Can you work these out from the model? Positions are in its coordinate system, mm. A direction names the side the tool comes from. Round coordinates to 2 decimals unless told otherwise and drop trailing zeros. Loops run counter-clockwise (first coordinate to the right, second up) from the corner with the lowest first, then second, coordinate; pieces in that order, holes last. Notation, with made-up numbers: M -20,-38.75 L 29,-38.75 A10 cw 29,-28.75 Z; hole C 77,27 d3. An arc over 180 degrees is marked long. Return JSON: item names as keys, results as strings.
```python
from build123d import *

# Parameters (mm, degrees)
SKETCH2_R                             = 14
SKETCH2_R_2                           = 11
BOSS_EXTRUDE7_DEPTH                   = 15
SKETCH2_12_R                          = 11
BOSS_EXTRUDE10_DEPTH                  = 3
SKETCH2_9_R                           = 14
SKETCH2_9_R_2                         = 11
BOSS_EXTRUDE8_DEPTH                   = 20
SKETCH2_11_R                          = 11
SKETCH2_11_R_2                        = 8.75
BOSS_EXTRUDE9_DEPTH                   = 12.5
BOSS_EXTRUDE11_REACH                  = 119.015
BOSS_EXTRUDE11_END_RADIUS             = 14
BOSS_EXTRUDE11_DIRECTION_2_REACH      = 119.015
BOSS_EXTRUDE11_DIRECTION_2_END_RADIUS = 14
CUT_EXTRUDE6_DEPTH                    = 1.1
SKETCH13_R                            = 1.15
CUT_EXTRUDE7_DEPTH                    = 3
BOSS_EXTRUDE12_REACH                  = 119.21
SKETCH15_W                            = 3
SKETCH15_H                            = 9.5
FILLET1_R                             = 2


with BuildPart() as part:
    # Sketch2 → Boss-Extrude7 (new body)
    with BuildSketch(Plane(origin=(0, 0, 0), x_dir=(1, 0, 0), z_dir=(0, 1, 0))):
        with Locations(Location((-50, 3.220631283, 0), (0, 0, 270))):
            Circle(SKETCH2_R)
        with Locations(Location((-50, 3.220631283, 0), (0, 0, 270))):
            Circle(SKETCH2_R_2, mode=Mode.SUBTRACT)
    extrude(amount=BOSS_EXTRUDE7_DEPTH)

    # Sketch2<12> → Boss-Extrude10 (add)
    with BuildSketch(Plane(origin=(0, 0, 0), x_dir=(1, 0, 0), z_dir=(0, 1, 0))):
        with Locations(Location((-50, 3.220631283, 0), (0, 0, 270))):
            Circle(SKETCH2_12_R)
    extrude(amount=BOSS_EXTRUDE10_DEPTH)


with BuildPart() as body_2:
    # Sketch2<9> → Boss-Extrude8 (new body)
    with BuildSketch(Plane(origin=(0, 0, 0), x_dir=(1, 0, 0), z_dir=(0, 1, 0))):
        with Locations(Location((100, 3.220631283, 0), (0, 0, 270))):
            Circle(SKETCH2_9_R)
        with Locations(Location((100, 3.220631283, 0), (0, 0, 270))):
            Circle(SKETCH2_9_R_2, mode=Mode.SUBTRACT)
    extrude(amount=BOSS_EXTRUDE8_DEPTH)

    # Sketch2<11> → Boss-Extrude9 (add)
    with BuildSketch(Plane(origin=(0, 0, 0), x_dir=(1, 0, 0), z_dir=(0, 1, 0))):
        with Locations(Location((100, 3.220631283, 0), (0, 0, 270))):
            Circle(SKETCH2_11_R)
        with Locations(Location((100, 3.220631283, 0), (0, 0, 270))):
            Circle(SKETCH2_11_R_2, mode=Mode.SUBTRACT)
    extrude(amount=BOSS_EXTRUDE9_DEPTH)


    add(part.part)  # Boss-Extrude11 merges part
    # Boss-Extrude11: up to this cylinder (the profile starts outside it)
    boss_extrude11_end = Plane(origin=(-50, 0.212132, -3.220631283), z_dir=(0, -1, 0)) * Cylinder(BOSS_EXTRUDE11_END_RADIUS, 267.03, mode=Mode.PRIVATE)
    # Sketch3 → Boss-Extrude11 (add, up to the surface)
    with BuildSketch(Plane(origin=(0, 0, 0), x_dir=(0, 0, -1), z_dir=(1, 0, 0)), mode=Mode.PRIVATE) as boss_extrude11_sk1:
        Polygon((10.720631283, 0), (10.720631283, 15), (-4.279368717, 15), (-4.279368717, 0), (-1.279368717, 0), (-1.279368717, 12), (7.720631283, 12), (7.720631283, 0), align=None)
    boss_extrude11_tool1 = extrude(boss_extrude11_sk1.sketch, amount=-BOSS_EXTRUDE11_REACH, mode=Mode.PRIVATE) - boss_extrude11_end
    add(boss_extrude11_tool1.solids().sort_by_distance((0, 0.212132, -9.220631))[0])

    # Boss-Extrude11 direction 2: up to this cylinder (the profile starts outside it)
    boss_extrude11_direction_2_end = Plane(origin=(100, 0.212132, -3.220631283), z_dir=(0, -1, 0)) * Cylinder(BOSS_EXTRUDE11_DIRECTION_2_END_RADIUS, 267.03, mode=Mode.PRIVATE)
    # Sketch3 → Boss-Extrude11 direction 2 (add, up to the surface)
    with BuildSketch(Plane(origin=(0, 0, 0), x_dir=(0, 0, -1), z_dir=(1, 0, 0)), mode=Mode.PRIVATE) as boss_extrude11_direction_2_sk1:
        Polygon((10.720631283, 0), (10.720631283, 15), (-4.279368717, 15), (-4.279368717, 0), (-1.279368717, 0), (-1.279368717, 12), (7.720631283, 12), (7.720631283, 0), align=None)
    boss_extrude11_direction_2_tool1 = extrude(boss_extrude11_direction_2_sk1.sketch, amount=BOSS_EXTRUDE11_DIRECTION_2_REACH, mode=Mode.PRIVATE) - boss_extrude11_direction_2_end
    add(boss_extrude11_direction_2_tool1.solids().sort_by_distance((0, 0.212132, -9.220631))[0])

    # Sketch10 → Cut-Extrude6 (cut)
    with BuildSketch(Plane(origin=(0, 3, 0), x_dir=(1, 0, 0), z_dir=(0, 1, 0))):
        Polygon((-47.85, 11.358676665), (-48.925, 13.220631283), (-51.075, 13.220631283), (-52.15, 11.358676665), (-51.075, 9.496722047), (-48.925, 9.496722047), align=None)
        Polygon((-58.138045382, 5.37063128), (-60, 4.29563128), (-60, 2.14563128), (-58.138045382, 1.07063128), (-56.276090764, 2.14563128), (-56.276090764, 4.29563128), align=None)
        Polygon((-41.861954618, 5.37063128), (-43.723909236, 4.29563128), (-43.723909236, 2.14563128), (-41.861954618, 1.07063128), (-40, 2.14563128), (-40, 4.29563128), align=None)
        Polygon((-47.85, -4.917414098), (-48.925, -3.05545948), (-51.075, -3.05545948), (-52.15, -4.917414098), (-51.075, -6.779368717), (-48.925, -6.779368717), align=None)
    extrude(amount=-CUT_EXTRUDE6_DEPTH, mode=Mode.SUBTRACT)

    # Sketch13 → Cut-Extrude7 (cut)
    with BuildSketch(Plane(origin=(0, 3, 0), x_dir=(1, 0, 0), z_dir=(0, 1, 0))):
        with Locations(Location((-50, 11.35867667, 0), (0, 0, 270))):
            Circle(SKETCH13_R)
        with Locations(Location((-41.86195462, 3.22063128, 0), (0, 0, 270))):
            Circle(SKETCH13_R)
        with Locations(Location((-50, -4.9174141, 0), (0, 0, 270))):
            Circle(SKETCH13_R)
        with Locations(Location((-58.13804538, 3.22063128, 0), (0, 0, 270))):
            Circle(SKETCH13_R)
    extrude(amount=-CUT_EXTRUDE7_DEPTH, mode=Mode.SUBTRACT)

    # Sketch15 → Boss-Extrude12 (add, up to next)
    with BuildSketch(Plane.XY.offset(-7.720631283), mode=Mode.PRIVATE) as boss_extrude12_sk1:
        with Locations((-13.807045748, 7.25)):
            Rectangle(SKETCH15_W, SKETCH15_H)
    boss_extrude12_tool1 = extrude(boss_extrude12_sk1.sketch, amount=BOSS_EXTRUDE12_REACH, mode=Mode.PRIVATE) - body_2.part
    # Sketch15 → Boss-Extrude12 (add, up to next)
    with BuildSketch(Plane.XY.offset(-7.720631283), mode=Mode.PRIVATE) as boss_extrude12_sk2:
        with Locations((12.064318086, 7.25)):
            Rectangle(SKETCH15_W, SKETCH15_H)
    boss_extrude12_tool2 = extrude(boss_extrude12_sk2.sketch, amount=BOSS_EXTRUDE12_REACH, mode=Mode.PRIVATE) - body_2.part
    # Sketch15 → Boss-Extrude12 (add, up to next)
    with BuildSketch(Plane.XY.offset(-7.720631283), mode=Mode.PRIVATE) as boss_extrude12_sk3:
        with Locations((37.93568192, 7.25)):
            Rectangle(SKETCH15_W, SKETCH15_H)
    boss_extrude12_tool3 = extrude(boss_extrude12_sk3.sketch, amount=BOSS_EXTRUDE12_REACH, mode=Mode.PRIVATE) - body_2.part
    # Sketch15 → Boss-Extrude12 (add, up to next)
    with BuildSketch(Plane.XY.offset(-7.720631283), mode=Mode.PRIVATE) as boss_extrude12_sk4:
        with Locations((63.807045754, 7.25)):
            Rectangle(SKETCH15_W, SKETCH15_H)
    boss_extrude12_tool4 = extrude(boss_extrude12_sk4.sketch, amount=BOSS_EXTRUDE12_REACH, mode=Mode.PRIVATE) - body_2.part
    add(boss_extrude12_tool1.solids().sort_by_distance((-13.807046, 7.25, -7.720631))[0])
    add(boss_extrude12_tool2.solids().sort_by_distance((12.064318, 7.25, -7.720631))[0])
    add(boss_extrude12_tool3.solids().sort_by_distance((37.935682, 7.25, -7.720631))[0])
    add(boss_extrude12_tool4.solids().sort_by_distance((63.807046, 7.25, -7.720631))[0])

    # Fillet1
    fillet1_edges = [body_2.edges().sort_by_distance(p)[0] for p in [
        (-15.307045748, 7.25, 1.279368717),
        (-12.307045748, 7.25, 1.279368717),
        (-12.307045748, 7.25, -7.720631283),
        (-15.307045748, 7.25, -7.720631283),
        (13.564318086, 7.25, 1.279368717),
        (10.564318086, 7.25, 1.279368717),
        (13.564318086, 7.25, -7.720631283),
        (10.564318086, 7.25, -7.720631283),
        (36.43568192, 7.25, 1.279368717),
        (39.43568192, 7.25, 1.279368717),
        (39.43568192, 7.25, -7.720631283),
        (36.43568192, 7.25, -7.720631283),
        (62.307045754, 7.25, 1.279368717),
        (65.307045754, 7.25, 1.279368717),
        (65.307045754, 7.25, -7.720631283),
        (62.307045754, 7.25, -7.720631283),
    ]]
    fillet(fillet1_edges, radius=FILLET1_R)


solid = body_2.part
```
Q1. On a 3-axis mill with a long thin cutter (end or side, diameter ignored), from which of +Z, -Z, +X, -X, +Y, -Y can I reach the whole of each face in a straight line? I mean faces 1 (the flat face through (25, 12, -3)), 2 (the flat face through (24, 8, 4.279)), 3 (the flat face through (24, 7, -10.721)). Say none if no direction works.
Results:
{"face 1": "-Y", "face 2": "+Z, +Y, -Y", "face 3": "-Z, +Y, -Y"}
Q2. Suppose I cut it at A-A, the plane x = 100. Please give me the cut outline in (y, z), plus the area to 3 significant figures.
Results:
{"outline": "M 0,-17.22 L 20,-17.22 L 20,-14.22 L 12.5,-14.22 L 12.5,-11.97 L 0,-11.97 Z; M 0,5.53 L 12.5,5.53 L 12.5,7.78 L 20,7.78 L 20,10.78 L 0,10.78 Z", "area": "176 mm2"}
Q3. Suppose I cut it at B-B, the plane x = 56. Please give me the cut outline in (y, z).
Results:
{"outline": "M 0,-10.72 L 15,-10.72 L 15,4.28 L 0,4.28 L 0,1.28 L 12,1.28 L 12,-7.72 L 0,-7.72 Z"}
Q4. If I drill on line 1 along X through (y, z) = (14.5, -4); line 2 along X through (y, z) = (8.5, -10); line 3 along Z through (x, y) = (53, 5.75), over which ranges is the centre line in solid material (lowest first)?
Results:
{"line 1": "x = -63.98 to -60.97, -39.03 to 89.03, 110.97 to 113.98", "line 2": "x = -62.25 to -58.66, -41.34 to 94.47, 105.53 to 112.25", "line 3": "z = -10.72 to -7.72, 1.28 to 4.28"}
Q5. Suppose I cut it at C-C, the plane y = 9. State how many separate pieces and enclosed holes the cut face has, plus the area to 3 significant figures.
Results:
{"separate pieces": "1", "enclosed holes": "7", "area": "1,480 mm2"}
Q6. Suppose I cut it at D-D, the plane x = -46. Please give me the cut outline in (y, z), plus the area to 3 significant figures.
Results:
{"outline": "M 0,-16.64 L 15,-16.64 L 15,-13.47 L 3,-13.47 L 3,7.03 L 15,7.03 L 15,10.2 L 0,10.2 Z", "area": "157 mm2"}
Q7. I'm going to push flat-ended pins straight in: pin 1 Ø2 at (y, z) = (7.5, 5) entering from -X; pin 2 Ø5 at (y, z) = (10.5, 2.5) entering from -X; pin 3 Ø1.5 at (y, z) = (8, -2.5) entering from -X; pin 4 Ø5 at (y, z) = (4.5, -11) entering from +X. Where does each tip first touch, or does it pass through?
Results:
{"pin 1": "stops at x = -61.99", "pin 2": "stops at x = -63.62", "pin 3": "stops at x = -64", "pin 4": "stops at x = 112.97"}
